Geometry check sheet. Reference: the model listing, model coordinates, mm. A direction names the side the tool comes from. Give positions to 0.01 mm unless a question says otherwise; leave off trailing zeros. Write each loop counter-clockwise with the first axis right and the second up, starting at its lowest first coordinate (ties: lowest second). Pieces come first, ordered by that corner, then holes. Notation, with made-up numbers: (29.5, 74.25) -> (55.5, 74.25) arc R13 ccw to (55.5, 95.25) -> close; hole circle Ø11 at (30, -19.5). An arc over 180 degrees is marked (long way). Use a Markdown table: item, result. Add a question column.
from build123d import *

# Parameters (mm, degrees)
SKETCH1_W           = 100
SKETCH1_H           = 20
BOSS_EXTRUDE4_START = 75
SKETCH6_R           = 25
BOSS_EXTRUDE4_DEPTH = 50


with BuildPart() as part:
    # Sketch1 → Revolve1 (revolve)
    with BuildSketch(Plane.YZ, mode=Mode.PRIVATE) as revolve1_sk:
        with Locations((50, 10)):
            Rectangle(SKETCH1_W, SKETCH1_H)
    revolve(revolve1_sk.sketch.rotate(Axis((0, 100, 0), (0, 0, 1)), 270), axis=Axis((0, 100, 0), (0, 0, 1)))

    # Sketch6 → Boss-Extrude4 (add)
    with BuildSketch(Plane(origin=(0, 0, 0), x_dir=(-1, 0, 0), z_dir=(0, 1, 0)).offset(BOSS_EXTRUDE4_START)):
        with BuildLine():
            Line((40, 20), (-40, 20))
            Line((-40, 20), (-40, 223))
            ThreePointArc((-40, 223), (0, 263), (40, 223))
            Line((40, 223), (40, 20))
        make_face()
        with Locations(Location((0, 222.24, 0), (0, 0, 90))):
            Circle(SKETCH6_R, mode=Mode.SUBTRACT)
    extrude(amount=BOSS_EXTRUDE4_DEPTH)


solid = part.part
1) Sectioned sample at B-B, the plane y = 100. Enter the section's corners in (x, z), and give its area (3 significant figures).
2) Sectioned sample at C-C, the plane z = 153.5. Enter the section's corners in (x, y), and give its area (3 significant figures).
3) Tool access check on faces 5 (the face through (40, 100, 120)), 6 (the face through (-1, 125, 143)), 7 (the face through (-40, 100, 123)). Record the directions out of +Z, -Z, +X, -X, +Y, -Y that give a thin tool (end or side, any length) a straight path to the whole face; none if there is none.
4) Gauge pin test, flat ends, axial feed: P1, Ø6, axis at x = 18, z = 160, coming from the +Y side; P2, Ø3, axis at x = -34, y = 21, coming from the +Z side; P3, Ø25, axis at y = 87.5, z = 157.5, coming from the -X side. Record the tip position at first contact, or that the pin passes through.
5) Sectioned sample at A-A, the plane x = 0. Enter the section's corners in (y, z).
6) Sectioned sample at D-D, the plane x = -49.5. Enter the section's corners in (y, z).
7) Material ranges on probe 1 along X at (y, z) = (104, 222); probe 2 along Z at (x, y) = (-47.5, 90); probe 3 along X at (y, z) = (122, 91), recorded low to high. Write a range as [from, to].
8) Draft check along Z on faces 1 (the face through (0.88, 99.65, 262.99)), 2 (the face through (-1, 75, 143)), 3 (the face through (1.099, 99.65, 197.264)), 4 (the face through (1, 99, 0)). Enter one of: +Z half, -Z half, draft (parallel to the pull), parting line (faces both ways), or undercut.
Check values:
| question | item | result |
|---|---|---|
| 1 | outline | (-100, 0) -> (100, 0) -> (100, 20) -> (40, 20) -> (40, 223) arc R40 ccw to (-40, 223) -> (-40, 20) -> (-100, 20) -> close; hole circle Ø50 at (0, 222.24) |
| 1 | area | 20,800 mm² |
| 2 | outline | (-40, 75) -> (40, 75) -> (40, 125) -> (-40, 125) -> close |
| 2 | area | 4,000 mm² |
| 3 | face 5 | +Z, +X, +Y, -Y |
| 3 | face 6 | +Z, +X, -X, +Y |
| 3 | face 7 | +Z, -X, +Y, -Y |
| 4 | P1 | y = 125 |
| 4 | P2 | z = 20 |
| 4 | P3 | x = -40 |
| 5 | outline | (0, 0) -> (200, 0) -> (200, 20) -> (125, 20) -> (125, 197.24) -> (75, 197.24) -> (75, 20) -> (0, 20) -> close; (75, 247.24) -> (125, 247.24) -> (125, 263) -> (75, 263) -> close |
| 6 | outline | (13.11, 0) -> (186.89, 0) -> (186.89, 20) -> (13.11, 20) -> close |
| 7 | probe 1 | [-40, -25], [25, 40] |
| 7 | probe 2 | [0, 20] |
| 7 | probe 3 | [-40, 40] |
| 8 | face 1 | +Z half |
| 8 | face 2 | draft |
| 8 | face 3 | undercut |
| 8 | face 4 | -Z half |
